Check sheet for the modelled part. Datum: model origin and axes. Units: mm. A direction names the side the tool comes from. Round coordinates to 2 decimals unless told otherwise and drop trailing zeros. Write each loop counter-clockwise with the first axis right and the second up, starting at its lowest first coordinate (ties: lowest second). Pieces come first, ordered by that corner, then holes. Notation, with made-up numbers: M -5,86.25 L 51,86.25 A24 ccw 51,111.25 Z; hole C 76,22 d2. An arc over 180 degrees is marked long. Put each result on its own line as item: value.
```python
from build123d import *

# Parameters (mm, degrees)
SKETCH1_R           = 1.54
SKETCH1_R_2         = 2.443409063
SKETCH1_R_3         = 0.85
SKETCH1_R_4         = 0.425
BOSS_EXTRUDE1_DEPTH = 1.6


with BuildPart() as part:
    # Sketch1 → Boss-Extrude1 (new body)
    with BuildSketch(Plane(origin=(0, 0, 0), x_dir=(1, 0, 0), z_dir=(0, 1, 0))):
        Polygon((2.07, 0), (2.07, -2.45), (0, -2.45), (0, -21.3), (3.1, -21.3), (3.1, -25.4), (0, -25.4), (-2.45, -25.4), (0, -42.2), (4.6, -47.12), (22, -47.12), (26.6, -42.2), (29.05, -25.4), (26.6, -25.4), (23.5, -25.4), (23.5, -21.3), (26.6, -21.3), (26.6, -2.5), (24.65, -2.5), (24.65, 0), (9.15, 0), (9.15, -2.5), (7.25, -2.5), (7.25, 0), align=None)
        with Locations(Location((22.51, -28.768011283, 0), (0, 0, 270))):
            Circle(SKETCH1_R, mode=Mode.SUBTRACT)
        with Locations(Location((4.19, -28.768011283, 0), (0, 0, 270))):
            Circle(SKETCH1_R, mode=Mode.SUBTRACT)
        with Locations(Location((13.451347261, -30.276590937, 0), (0, 0, 270))):
            Circle(SKETCH1_R_2, mode=Mode.SUBTRACT)
        with Locations(Location((13.3, -7.22, 0), (0, 0, 270))):
            Circle(SKETCH1_R_3, mode=Mode.SUBTRACT)
        with Locations(Location((13.3, -17.92, 0), (0, 0, 270))):
            Circle(SKETCH1_R_3, mode=Mode.SUBTRACT)
        with Locations(Location((13.3, -3.2, 0), (0, 0, 270))):
            Circle(SKETCH1_R_4, mode=Mode.SUBTRACT)
        with Locations(Location((15.7, -3.2, 0), (0, 0, 270))):
            Circle(SKETCH1_R_4, mode=Mode.SUBTRACT)
        with Locations(Location((10.9, -3.2, 0), (0, 0, 270))):
            Circle(SKETCH1_R_4, mode=Mode.SUBTRACT)
        with Locations(Location((4, -14.97, 0), (0, 0, 270))):
            Circle(SKETCH1_R_4, mode=Mode.SUBTRACT)
        with Locations(Location((4, -12.57, 0), (0, 0, 270))):
            Circle(SKETCH1_R_4, mode=Mode.SUBTRACT)
        with Locations(Location((4, -10.17, 0), (0, 0, 270))):
            Circle(SKETCH1_R_4, mode=Mode.SUBTRACT)
        Polygon((20.7, -19.32), (20.7, -17.32), (19.75, -17.32), (19.75, -18), (17.8, -18), (17.8, -19.32), align=None, mode=Mode.SUBTRACT)
        Polygon((8.8, -19.32), (5.9, -19.32), (5.9, -17.32), (6.85, -17.32), (6.85, -18), (8.8, -18), align=None, mode=Mode.SUBTRACT)
        Polygon((17.8, -5.82), (20.7, -5.82), (20.7, -7.82), (19.75, -7.82), (19.75, -7.14), (17.8, -7.14), align=None, mode=Mode.SUBTRACT)
        Polygon((5.9, -5.82), (5.9, -7.82), (6.85, -7.82), (6.85, -7.14), (8.8, -7.14), (8.8, -5.82), align=None, mode=Mode.SUBTRACT)
    extrude(amount=BOSS_EXTRUDE1_DEPTH)


solid = part.part
```
1. Cross-section at C-C (z = 33.5). Enter the section's corners in (x, y), then the cut area to 3 significant figures.
Computed values:
outline: M -1.27,0 L 27.87,0 L 27.87,1.6 L -1.27,1.6 Z
area: 46.6 mm2
2. Depth check by flat-ended pin: pin 1 Ø1.5 at (x, z) = (14.5, 21.5) entering from -Y; pin 2 Ø0.8 at (y, z) = (1, 1) entering from +X; pin 3 Ø0.5 at (y, z) = (1, 12.5) entering from -X. Enter the tip coordinate at first touch or a pass-through.
Computed values:
pin 1: stops at y = 0
pin 2: stops at x = 24.65
pin 3: stops at x = 0
3. Cross-section at A-A (x = 25.5). Enter the section's corners in (y, z).
Computed values:
outline: M 0,2.5 L 1.6,2.5 L 1.6,21.3 L 0,21.3 Z; M 0,25.4 L 1.6,25.4 L 1.6,43.38 L 0,43.38 Z
4. Cross-section at B-B (y = 0.8). Count the separate pieces of the cut face and the enclosed holes in it, then the cut area to 3 significant figures.
Computed values:
separate pieces: 1
enclosed holes: 15
area: 1,170 mm2
5. Scan lines: probe 1 along Z at (x, y) = (7, 0.8); probe 2 along Z at (x, y) = (8, 1.15); probe 3 along Z at (x, y) = (14, 0.2). Record each from-to range of solid material in increasing order.
Computed values:
probe 1: z = 0 to 5.82, 7.14 to 18, 19.32 to 47.12
probe 2: z = 2.5 to 5.82, 7.14 to 18, 19.32 to 47.12
probe 3: z = 0 to 6.74, 7.7 to 17.44, 18.4 to 27.9, 32.66 to 47.12
6. Access from +Z, -Z, +X, -X, +Y, -Y to the whole of each face (thin tool, end or side, straight path). Record for faces 4 (the flat face through (23.5, 1, 23)), 5 (the flat face through (3.1, 1, 23)), 6 (the flat face through (8, 1, 7.14)).
Computed values:
face 4: +X, +Y, -Y
face 5: -X, +Y, -Y
face 6: +Y, -Y
7. Release check for a two-part mould opening along X. For faces 1 (the flat face through (24.65, 1, 1)), 2 (the flat face through (0, 1, 12)), 3 (the flat face through (7, 1, 19.32)) record: +X half, -X half, draft (parallel to the pull), parting line (faces both ways), or undercut.
Computed values:
face 1: +X half
face 2: -X half
face 3: undercut
